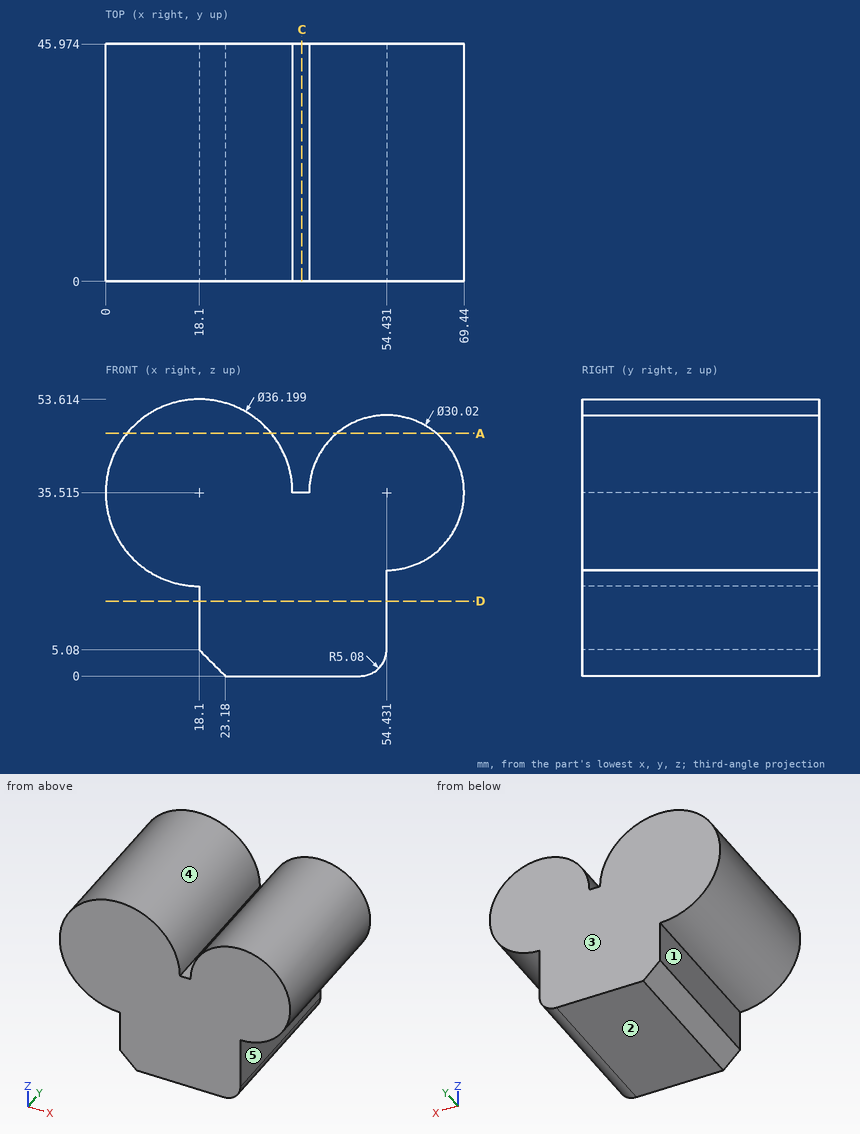
The figure shows three views and two pictorial views of one solid part (mm, origin at its lowest corner). Answer the questions. A direction names the side the tool comes from. Give positions to 0.01 mm unless a question says otherwise; leave off trailing zeros. Loops run counter-clockwise (first coordinate to the right, second up) from the corner with the lowest first, then second, coordinate; pieces in that order, holes last. Notation, with made-up numbers: (87, 52.5) -> (143, 52.5) arc R22 ccw to (143, 69.5) -> close; hole circle Ø9 at (-31, 41). An arc over 180 degrees is marked (long way). Put each result on its own line as item: value. Start each with the question number.
Item 1: Each of these flat-tipped pins is pushed along its axis until it touches: P1, Ø4.5, axis at y = 11.5, z = 15.5, coming from the +X side; P2, Ø3, axis at x = 41, y = 6.5, coming from the +Z side (1 decimal); P3, Ø6, axis at y = 28, z = 11.5, coming from the -X side. Where does it stop, or does it pass through?
Item 2: Which of the six approach directions +Z, -Z, +X, -X, +Y, -Y give full straight-line access (tool end or side, diameter ignored) to the marked faces 1 and 2?
Item 3: The mould has two halves that part along X. Classify the marked faces 3, 4 and 5: released by +X, released by -X, zero draft, split by the parting line, or undercut.
Item 4: The part is cut by section C-C (x = 38). Give the vertices of the cut face in (y, z) (1 decimal).
Item 5: The part is cut by section A-A (z = 47). Give the vertices of the cut face in (x, y) (1 decimal).
Item 6: The part is cut by section D-D (z = 14.5). Give the vertices of the cut face in (x, y).
Item 7: Find the intervals of material crossed by L1, parallel to X at y = 41, z = 5.5; L2, parallel to X at y = 31, z = 41; L3, parallel to X at y = 28, z = 4 (1 decimal), in increasing order. Write a range as [from, to].
Answers below:
1. P1: x = 54.43
1. P2: z = 44.6
1. P3: x = 18.1
2. face 1: -Z, -X, +Y, -Y
2. face 2: -Z, +X, -X, +Y, -Y
3. face 3: zero draft
3. face 4: undercut
3. face 5: released by +X
4. outline: (0, 0) -> (46, 0) -> (46, 35.5) -> (0, 35.5) -> close
5. outline: (4.1, 0) -> (32.1, 0) -> (32.1, 46) -> (4.1, 46) -> close; (44.8, 0) -> (64.1, 0) -> (64.1, 46) -> (44.8, 46) -> close
6. outline: (18.1, 0) -> (54.43, 0) -> (54.43, 45.97) -> (18.1, 45.97) -> close
7. L1: [18.1, 54.43]
7. L2: [0.85, 35.35], [40.46, 68.4]
7. L3: [19.2, 54.3]
